Input: part model. Units: mm. Frame: model coordinates. Face numbers are marked on the shaded views. Coordinates: 2 decimals unless noted, no trailing zeros. Order: outer loops, then holes, each group sorted by start corner. A loop starts at its lowest first (then second) coordinate and runs counter-clockwise, first axis right, second up. Notation, with made-up numbers: (18, -17.5) -> (45, -17.5) arc R19 cw to (45, -2.5) -> close; hole circle Ø5 at (77.5, 3). An arc over 180 degrees is marked (long way). One line per question, with ' | ' between items.
```python
from build123d import *

# Parameters (mm, degrees)
F0_W           = 180
F0_H           = 200
F1_DEPTH       = 10
F2_D           = 5.5
F2_CBORE_D     = 9.75
F2_CBORE_DEPTH = 5
F4_D           = 5.5
F4_CBORE_D     = 9.75
F4_CBORE_DEPTH = 5
F6_D           = 4


with BuildPart() as f1:
    # F0 (on Front) → F1 (new body)
    with BuildSketch(Plane.XZ):
        Rectangle(F0_W, F0_H)
    extrude(amount=F1_DEPTH)

    # F2 (through all)
    with Locations(Plane(origin=(0, 0, 0), x_dir=(1, 0, 0), z_dir=(0, 1, 0))):
        with Locations((-45, -62.5), (-20, -62.5), (-20, -37.5), (-45, -37.5), (20, -62.5), (45, -62.5), (45, -37.5), (20, -37.5), (12.5, 37.5), (-12.5, 37.5), (-12.5, 62.5), (12.5, 62.5)):
            CounterBoreHole(F2_D / 2, F2_CBORE_D / 2, F2_CBORE_DEPTH)

    # F4 (through all)
    with Locations(Plane.XZ.offset(10)):
        with Locations((-62.5, -37.5), (-62.5, -12.5), (-37.5, -12.5), (-37.5, -37.5), (-62.5, 27.5), (-62.5, 52.5), (-37.5, 52.5), (-37.5, 27.5), (37.5, -1), (37.5, 24), (62.5, 24), (62.5, -1)):
            CounterBoreHole(F4_D / 2, F4_CBORE_D / 2, F4_CBORE_DEPTH)

    # F6 (through all)
    with Locations(Plane.XZ.offset(10)):
        with Locations((-17.5, 12), (-17.5, -12), (17.5, -12), (17.5, 12), (-12, 17.5), (12, 17.5), (12, -17.5), (-12, -17.5)):
            Hole(F6_D / 2)


solid = f1.part
```
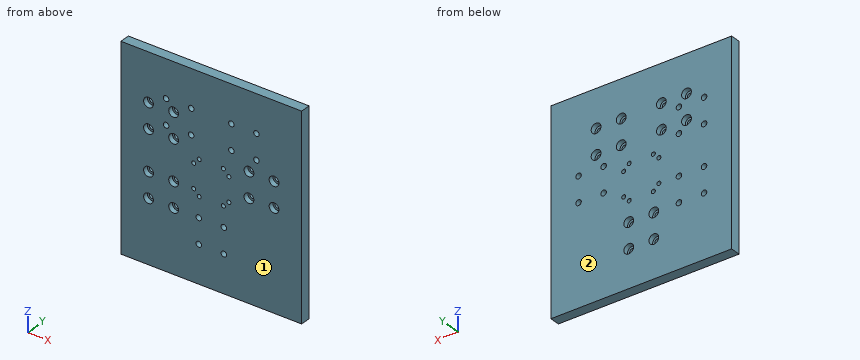
1. Mould query, pull axis Y, two halves, no side actions, for the marked faces 1 and 2. Classes: released by +Y, released by -Y, zero draft, split by the parting line, or undercut.
Recorded:
face 1: released by -Y | face 2: released by +Y
2. Ray query, line 1 (Z direction, x = 41, y = -1.75); line 2 (Z direction, x = -62.5, y = -3.15); line 3 (Z direction, x = 12, y = -9.25). Return the intervals inside material, ascending. Write a range as [from, to].
Recorded:
line 1: z = [-100, 34.71], [40.29, 59.71], [65.29, 100] | line 2: z = [-100, -40.25], [-34.75, -15.25], [-9.75, 24.75], [30.25, 49.75], [55.25, 100] | line 3: z = [-100, -65.2], [-59.8, -40.2], [-34.8, -19.5], [-15.5, 15.5], [19.5, 100]
3. Cut plane B-B, the plane z = 37.5. State how many separate pieces and enclosed holes the cut face has, and give its area (4 significant figures).
Recorded:
separate pieces: 5 | enclosed holes: 0 | area: 1,495 mm^2
4. Pin query (flat end, axial travel): pin 1 Ø5 at (x, z) = (-40, -13.5) entering from -Y; pin 2 Ø5 at (x, z) = (14, -39) entering from +Y. Return the tip coordinate at first contact, or that it passes through.
Recorded:
pin 1: stops at y = -10 | pin 2: stops at y = -5
5. Cut plane A-A, the plane x = 45. Return loops of the section in (y, z) (3 decimals), and give its area (3 significant figures).
Recorded:
outline: (-10, -100) -> (0, -100) -> (0, 32.625) -> (-5, 32.625) -> (-5, 34.75) -> (-10, 34.75) -> close; (-10, 40.25) -> (-5, 40.25) -> (-5, 42.375) -> (0, 42.375) -> (0, 57.625) -> (-5, 57.625) -> (-5, 59.75) -> (-10, 59.75) -> close; (-10, 65.25) -> (-5, 65.25) -> (-5, 67.375) -> (0, 67.375) -> (0, 100) -> (-10, 100) -> close | area: 1,850 mm^2
